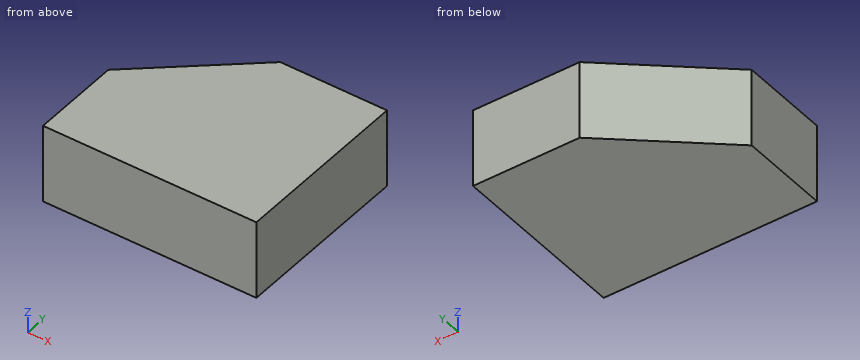
from build123d import *

# Parameters (mm, degrees)
SKETCH1_W          = 13.648457072
SKETCH1_H          = 11.499915192
EXTRUDE1_DEPTH     = 2.5
CUT_EXTRUDE1_DEPTH = 10


with BuildPart() as part:
    # Sketch1 → Extrude1 (new, symmetric)
    with BuildSketch(Plane.XY):
        with Locations((6.824228536, 5.749957596)):
            Rectangle(SKETCH1_W, SKETCH1_H)
    extrude(amount=EXTRUDE1_DEPTH, both=True)

    # Sketch2 → Cut-Extrude1 (cut)
    with BuildSketch(Plane(origin=(0, 0, -2.5), x_dir=(-1, 0, 0), z_dir=(0, 0, -1))):
        Polygon((-6.824228536, 11.499915192), (0, 5.749957596), (0, 11.499915192), align=None)
    extrude(amount=-CUT_EXTRUDE1_DEPTH, mode=Mode.SUBTRACT)


solid = part.part
Verification items for the finished model (mm, model axes). Give positions to 0.01 mm unless a question says otherwise; leave off trailing zeros. Write each loop counter-clockwise with the first axis right and the second up, starting at its lowest first coordinate (ties: lowest second). Pieces come first, ordered by that corner, then holes.
(1) Cross-section at C-C (x = 4.5). Enter the section's corners in (y, z), plus the area to 3 significant figures.
(2) Cross-section at B-B (x = 2.5). Enter the section's corners in (y, z), plus the area to 3 significant figures.
(3) Gauge pin test, flat end, axial feed: pin 1 (2 mm diameter, centred on x = 5, z = 0, fed in from +Y). Record the tip position at first contact, or that the pin passes through.
(4) Material ranges on line 1 (X direction, y = 6.25, z = 1.8); line 2 (Y direction, x = 4, z = 1.6); line 3 (X direction, y = 8.75, z = -0.85), recorded low to high.
(5) Cross-section at A-A (z = -1.1). Enter the section's corners in (x, y).
Worked out:
1. outline: (0, -2.5) - (9.54, -2.5) - (9.54, 2.5) - (0, 2.5) - close
1. area: 47.7 mm2
2. outline: (0, -2.5) - (7.86, -2.5) - (7.86, 2.5) - (0, 2.5) - close
2. area: 39.3 mm2
3. pin 1: stops at y = 10.81
4. line 1: x = 0.59 to 13.65
4. line 2: y = 0 to 9.12
4. line 3: x = 3.56 to 13.65
5. outline: (0, 0) - (13.65, 0) - (13.65, 11.5) - (6.82, 11.5) - (0, 5.75) - close
